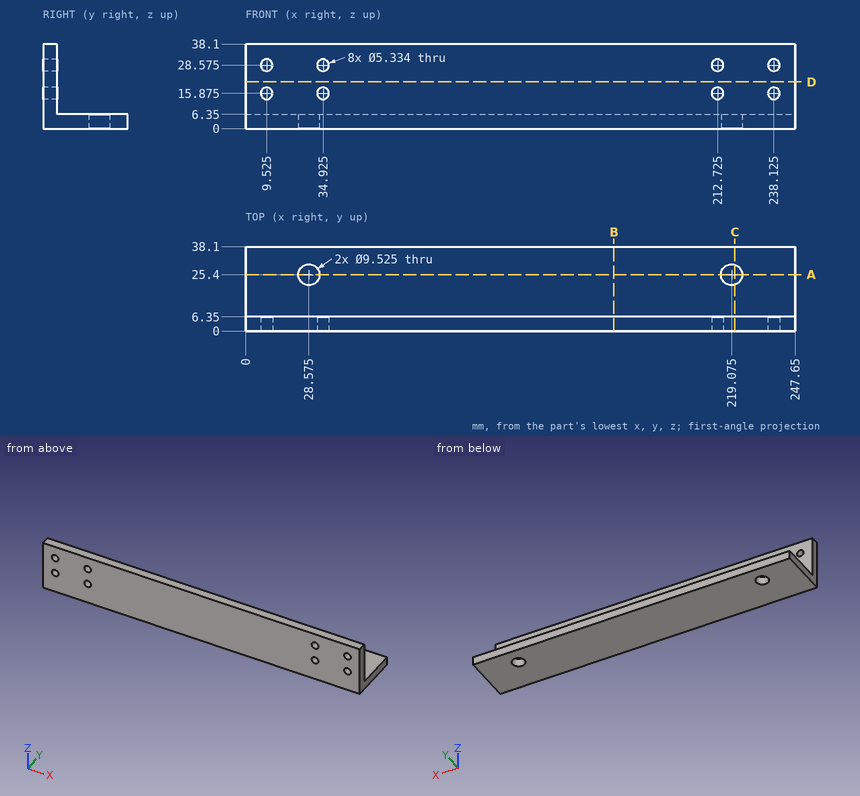
Input: dimensioned drawing with shaded views. Units: mm. Origin: part minimum x, y, z. Coordinates: 2 decimals unless noted, no trailing zeros. Order: outer loops, then holes, each group sorted by start corner. A loop starts at its lowest first (then second) coordinate and runs counter-clockwise, first axis right, second up. Notation, with made-up numbers: M 84,32 L 90,32 A31 cw 90,59 Z; hole C -16.5,-36.75 d3. An arc over 180 degrees is marked long. Answer as CSV lines item,"result".
Q1. Line query: probe 1 along Z at (x, y) = (213.5, 3); probe 2 along Z at (x, y) = (103, 9.5). Output: solid intervals per line, ascending. Write a range as [from, to].
Answers:
probe 1,"z = [0, 13.32], [18.43, 26.02], [31.13, 38.1]"
probe 2,"z = [0, 6.35]"
Q2. Section A-A on y = 25.4. Return the cut outline in (x, z).
Answers:
outline,"M 0,0 L 23.81,0 L 23.81,6.35 L 0,6.35 Z; M 33.34,0 L 214.31,0 L 214.31,6.35 L 33.34,6.35 Z; M 223.84,0 L 247.65,0 L 247.65,6.35 L 223.84,6.35 Z"
Q3. Section D-D on z = 21. Return the cut outline in (x, y), and give its area (3 significant figures).
Answers:
outline,"M 0,0 L 247.65,0 L 247.65,6.35 L 0,6.35 Z"
area,"1,570 mm^2"
Q4. Section C-C on x = 220.5. Return the cut outline in (y, z), and give its area (3 significant figures).
Answers:
outline,"M 0,0 L 20.86,0 L 20.86,6.35 L 6.35,6.35 L 6.35,38.1 L 0,38.1 Z; M 29.94,0 L 38.1,0 L 38.1,6.35 L 29.94,6.35 Z"
area,"386 mm^2"
Q5. First-contact query: P1, Ø1, axis at x = 137.5, z = 11.5, coming from the -Y side; P2, Ø8.5, axis at x = 212.725, z = 28.575, coming from the +Y side; P3, Ø10, axis at x = 97, y = 33, coming from the +Z side. Flat tips, straight axial feed; report the tip coordinate or a pass-through.
Answers:
P1,"stops at y = 0"
P2,"stops at y = 6.35"
P3,"stops at z = 6.35"
Q6. Section B-B on x = 166. Return the cut outline in (y, z).
Answers:
outline,"M 0,0 L 38.1,0 L 38.1,6.35 L 6.35,6.35 L 6.35,38.1 L 0,38.1 Z"
